The listing builds one solid part. Answer for the finished solid, in the listing's coordinates (mm). Face numbers are marked on the shaded views. A direction names the side the tool comes from. Give positions to 0.01 mm unless a question says otherwise; leave off trailing zeros. Order: outer loops, then holes, each group sorted by start corner. A loop starts at its lowest first (then second) coordinate and runs counter-clockwise, first axis right, second up.
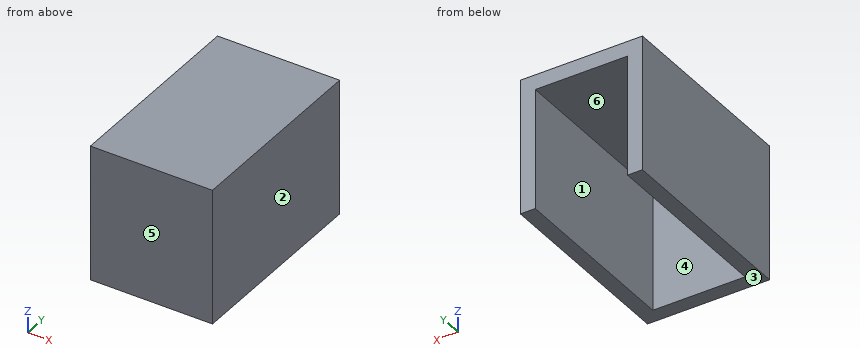
```python
from build123d import *

# Parameters (mm, degrees)
EXTRUDE_1_DEPTH = 16.2
SKETCH_4_W      = 16.4
SKETCH_4_H      = 26.4
EXTRUDE_2_DEPTH = 2


with BuildPart() as part:
    # 草图1 → 凸台-拉伸1 (new body)
    with BuildSketch(Plane.XY):
        Polygon((-8.004506799, -8.377067037), (-8.004506799, 14.022932963), (-8.004506799, 16.022932963), (-10.004506799, 16.022932963), (-10.004506799, 14.022932963), (-10.004506799, -10.377067037), (6.395493201, -10.377067037), (6.395493201, 14.022932963), (6.395493201, 16.022932963), (4.395493201, 16.022932963), (4.395493201, 14.022932963), (4.395493201, -8.377067037), align=None)
    extrude(amount=EXTRUDE_1_DEPTH)

    # 草图4 → 凸台-拉伸2 (add)
    with BuildSketch(Plane.XY.offset(16.2)):
        with Locations((-1.804506799, 2.822932963)):
            Rectangle(SKETCH_4_W, SKETCH_4_H)
    extrude(amount=EXTRUDE_2_DEPTH)


solid = part.part
```
1) Find section C-C (x = -3.75). Write down the section's boundary in (y, z).
Geometry says:
outline: (-10.38, 0) - (-8.38, 0) - (-8.38, 16.2) - (16.02, 16.2) - (16.02, 18.2) - (-10.38, 18.2) - close
2) A tool of negligible diameter and unlimited length cuts with its end or side. For the marked faces 5 and 6, from which of +Z, -Z, +X, -X, +Y, -Y can it reach the whole face along a straight path? Write none if from no direction.
Geometry says:
face 5: +Z, -Z, +X, -X, -Y
face 6: -Z, +Y
3) Straight lines are drawn through the part: probe 1 along X at (y, z) = (2.5, 7.75); probe 2 along Y at (x, z) = (-7.5, 13.5); probe 3 along Z at (x, y) = (3.5, 14). For each, find the intervals that lie inside material, in ascending order.
Geometry says:
probe 1: x = -10 to -8, 4.4 to 6.4
probe 2: y = -10.38 to -8.38
probe 3: z = 16.2 to 18.2
4) Find section A-A (y = 4.5). Write down the section's boundary in (x, z).
Geometry says:
outline: (-10, 0) - (-8, 0) - (-8, 16.2) - (4.4, 16.2) - (4.4, 0) - (6.4, 0) - (6.4, 18.2) - (-10, 18.2) - close
5) Given P1, Ø6, axis at x = -1, y = 9, coming from the -Z side; P2, Ø1.5, axis at x = -0.5, z = 14, coming from the +Y side, each flat-ended and moving along its own axis, determine where each tip first touches the part or whether it passes through.
Geometry says:
P1: stops at z = 16.2
P2: stops at y = -8.38
6) For a pull along X with two mould halves and no side action, classify the marked faces 1, 2, 3 and 4 as +X half, -X half, draft (parallel to the pull), parting line (faces both ways), or undercut.
Geometry says:
face 1: undercut
face 2: +X half
face 3: draft
face 4: undercut
7) Find section B-B (z = 4). Write down the section's boundary in (x, y).
Geometry says:
outline: (-10, -10.38) - (6.4, -10.38) - (6.4, 16.02) - (4.4, 16.02) - (4.4, -8.38) - (-8, -8.38) - (-8, 16.02) - (-10, 16.02) - close
